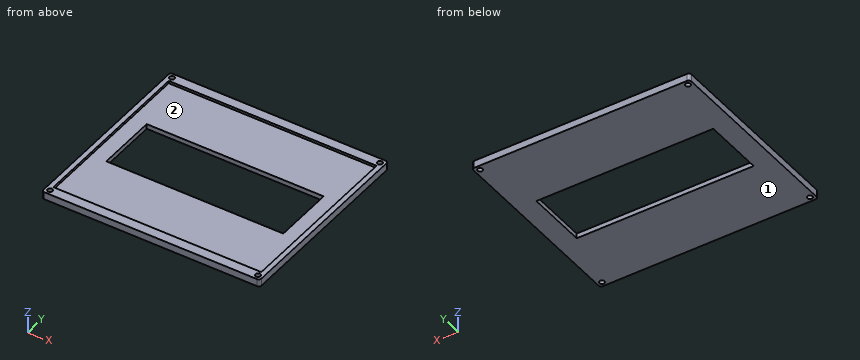
```python
from build123d import *

# Parameters (mm, degrees)
SKETCH2_W           = 88
SKETCH2_H           = 78
BOSS_EXTRUDE1_DEPTH = 3
SKETCH3_W           = 84
SKETCH3_H           = 70
CUT_EXTRUDE1_DEPTH  = 1
SKETCH4_R           = 1
CUT_EXTRUDE2_DEPTH  = 3
FILLET1_R           = 1
SKETCH5_W           = 71.5
SKETCH5_H           = 24.5
CUT_EXTRUDE3_DEPTH  = 3


with BuildPart() as part:
    # Sketch2 → Boss-Extrude1 (new body)
    with BuildSketch(Plane.XY):
        Rectangle(SKETCH2_W, SKETCH2_H)
    extrude(amount=BOSS_EXTRUDE1_DEPTH)

    # Sketch3 → Cut-Extrude1 (cut)
    with BuildSketch(Plane.XY.offset(3)):
        Rectangle(SKETCH3_W, SKETCH3_H)
    extrude(amount=-CUT_EXTRUDE1_DEPTH, mode=Mode.SUBTRACT)

    # Sketch4 → Cut-Extrude2 (cut)
    with BuildSketch(Plane.XY.offset(3)):
        with Locations((-42, 37)):
            Circle(SKETCH4_R)
        with Locations((42, 37)):
            Circle(SKETCH4_R)
        with Locations((-42, -37)):
            Circle(SKETCH4_R)
        with Locations((42, -37)):
            Circle(SKETCH4_R)
    extrude(amount=-CUT_EXTRUDE2_DEPTH, mode=Mode.SUBTRACT)

    # Fillet1
    fillet1_edges = [part.edges().sort_by_distance(p)[0] for p in [
        (-44, -39, 1.5),
        (-44, 39, 1.5),
        (44, 39, 1.5),
        (44, -39, 1.5),
    ]]
    fillet(fillet1_edges, radius=FILLET1_R)

    # Sketch5 → Cut-Extrude3 (cut)
    with BuildSketch(Plane.XY.offset(2)):
        Rectangle(SKETCH5_W, SKETCH5_H)
    extrude(amount=-CUT_EXTRUDE3_DEPTH, mode=Mode.SUBTRACT)


solid = part.part
```
Design review of the part built by this model. Coordinates are the model's own, in mm. Face numbers are marked on the shaded views. Coordinates: 2 decimals unless noted, no trailing zeros. Loops run counter-clockwise (first coordinate to the right, second up) from the corner with the lowest first, then second, coordinate; pieces in that order, holes last. Notation, with made-up numbers: (72.5, 50.5) - (128.5, 50.5) arc R9 cw to (128.5, 54.5) - close; hole circle Ø11 at (13, 46.5). An arc over 180 degrees is marked (long way). Use CSV: the item, a comma, the result in double quotes. Start each with the question number.
1) For pin 1 Ø3 at (x, y) = (30.5, 28.5) entering from +Z, flat-tipped, find the tip position at first contact; note if it passes through.
2) Consider section D-D on y = -37. Write out the cut boundary in (x, z), then the cut area to 3 significant figures.
3) Consider section A-A on x = -6.5. Write out the cut boundary in (y, z), then the cut area to 3 significant figures.
4) The part is to be moulded in two halves that separate along X. For the marked faces 1 and 2, say which applies: +X half, -X half, draft (parallel to the pull), parting line (faces both ways), or undercut.
5) Consider section B-B on z = 0.7. Write out the cut boundary in (x, y), then the cut area to 3 significant figures.
6) Wall thickness on L1, parallel to Y at x = 42, z = 1.35; L2, parallel to Y at x = 29, z = 1.15; L3, parallel to X at y = 18.5, z = 2.25: over which ranges is each line inside the solid? List them lowest first. Write a range as from..to.
7) Consider section C-C on y = -10. Write out the cut boundary in (x, z).
Geometry says:
1,pin 1,"z = 2"
2,outline,"(-44, 0) - (-43, 0) - (-43, 3) - (-44, 3) - close; (-41, 0) - (41, 0) - (41, 3) - (-41, 3) - close; (43, 0) - (44, 0) - (44, 3) - (43, 3) - close"
2,area,"252 mm^2"
3,outline,"(-39, 0) - (-12.25, 0) - (-12.25, 2) - (-35, 2) - (-35, 3) - (-39, 3) - close; (12.25, 0) - (39, 0) - (39, 3) - (35, 3) - (35, 2) - (12.25, 2) - close"
3,area,"115 mm^2"
4,face 1,"draft"
4,face 2,"undercut"
5,outline,"(-44, -38) arc R1 ccw to (-43, -39) - (43, -39) arc R1 ccw to (44, -38) - (44, 38) arc R1 ccw to (43, 39) - (-43, 39) arc R1 ccw to (-44, 38) - close; hole circle Ø2 at (-42, -37); hole circle Ø2 at (-42, 37); hole (-35.75, -12.25) - (35.75, -12.25) - (35.75, 12.25) - (-35.75, 12.25) - close; hole circle Ø2 at (42, -37); hole circle Ø2 at (42, 37)"
5,area,"5,100 mm^2"
6,L1,"-39..-38, -36..36, 38..39"
6,L2,"-39..-12.25, 12.25..39"
6,L3,"-44..-42, 42..44"
7,outline,"(-44, 0) - (-35.75, 0) - (-35.75, 2) - (-42, 2) - (-42, 3) - (-44, 3) - close; (35.75, 0) - (44, 0) - (44, 3) - (42, 3) - (42, 2) - (35.75, 2) - close"
